Verification items for the finished model (mm, model axes). Give positions to 0.01 mm unless a question says otherwise; leave off trailing zeros. Write each loop counter-clockwise with the first axis right and the second up, starting at its lowest first coordinate (ties: lowest second). Pieces come first, ordered by that corner, then holes. Notation, with made-up numbers: (31.25, -34) -> (57.25, -34) arc R37 ccw to (57.25, 5) -> close; hole circle Ø10 at (71, 1.25). An arc over 180 degrees is marked (long way). Answer as CSV lines item,"result". Start each with the question number.
1) Mould release check, pull along Z, two halves, no side actions. Record for faces 1 (the flat face through (-6, -4, 178)), 2 (the cylindrical face through (-5.082, -5.34, 14.388)), 3 (the cylindrical face through (-0.517, 7.377, 150.747)), 4 (the flat face through (-6, -4, 0)): released by +Z, released by -Z, zero draft, split by the parting line, or undercut.
2) Sectioned sample at C-C on z = 56. Record the cut outline in (x, y).
3) Sectioned sample at B-B on z = 163. Record the cut outline in (x, y), and give its area (3 significant figures).
4) Material ranges on L1, parallel to Z at x = 0, y = 7.7; L2, parallel to Y at x = 0, z = 131.5; L3, parallel to X at y = 7.35, z = 163, recorded low to high.
5) Gauge pin test, flat ends, axial feed: pin 1 Ø6 at (y, z) = (0.5, 110.5) entering from -X; pin 2 Ø2 at (x, z) = (3.5, 119) entering from -Y; pin 3 Ø3 at (x, z) = (2, 37.5) entering from -Y. Record the tip position at first contact, or that the pin passes through.
6) Sectioned sample at A-A on y = 0. Record the cut outline in (x, z).
```python
from build123d import *

# Parameters (mm, degrees)
SKETCH1_R               = 8
SKETCH1_R_2             = 6.9
BOSS_EXTRUDE1_DEPTH     = 163
SKETCH3_R               = 8
SKETCH3_R_2             = 6.9
BOSS_EXTRUDE3_DEPTH     = 15
CUT_EXTRUDE1_DEPTH      = 179.359188157
CUT_EXTRUDE1_DEPTH_BACK = 179.359188157
SKETCH2_R               = 1.6
SKETCH2_R_2             = 1.35
SKETCH4_R               = 1.4
CUT_EXTRUDE2_DEPTH      = 179.359188267
CIRPATTERN1_COUNT       = 2
CIRPATTERN1_ANGLE       = 90


with BuildPart() as part:
    # Sketch1 → Boss-Extrude1 (new body)
    with BuildSketch(Plane.XY):
        Circle(SKETCH1_R)
        Circle(SKETCH1_R_2, mode=Mode.SUBTRACT)
    extrude(amount=BOSS_EXTRUDE1_DEPTH)

    # Sketch3 → Boss-Extrude3 (add)
    with BuildSketch(Plane.XY.offset(163)):
        Circle(SKETCH3_R)
        Circle(SKETCH3_R_2, mode=Mode.SUBTRACT)
    extrude(amount=BOSS_EXTRUDE3_DEPTH)

    # Sketch2 → Cut-Extrude1 (cut, two sides: drawn at the far end of the back side and taken through both)
    with BuildSketch(Plane(origin=(0, 0, 0), x_dir=(1, 0, 0), z_dir=(0, 1, 0)).offset(-CUT_EXTRUDE1_DEPTH_BACK)):
        with Locations(Location((0, -163, 0), (0, 0, 270))):
            Circle(SKETCH2_R)
        with Locations(Location((0, -149.5, 0), (0, 0, 270))):
            Circle(SKETCH2_R_2)
    extrude(amount=CUT_EXTRUDE1_DEPTH + CUT_EXTRUDE1_DEPTH_BACK, mode=Mode.SUBTRACT)

    # Sketch4 → Cut-Extrude2 (cut, symmetric)
    with BuildSketch(Plane(origin=(0, 0, 0), x_dir=(0, 0, 1), z_dir=(0.7071067811865464, 0.7071067811865488, 0))):
        with Locations(Location((13, 0, 0), (0, 0, 270))):
            Circle(SKETCH4_R)
        with Locations(Location((5, 0, 0), (0, 0, 270))):
            Circle(SKETCH4_R)
    cut_extrude2 = extrude(amount=CUT_EXTRUDE2_DEPTH, both=True, mode=Mode.SUBTRACT)

    # CirPattern1: Cut-Extrude2 ×2 about axis
    cirpattern1_axis = Axis((0, 0, -8.9), (0, 0, 1))
    for i in range(1, CIRPATTERN1_COUNT):
        add(cut_extrude2.rotate(cirpattern1_axis, i * CIRPATTERN1_ANGLE / (CIRPATTERN1_COUNT - 1)), mode=Mode.SUBTRACT)


solid = part.part
```
Ans:
1,face 1,"released by +Z"
1,face 2,"undercut"
1,face 3,"undercut"
1,face 4,"released by -Z"
2,outline,"circle Ø16 at (0, 0); hole circle Ø13.8 at (0, 0)"
3,outline,"(-1.6, -7.84) -> (-1.6, -6.71) arc R6.9 cw to (-1.6, 6.71) -> (-1.6, 7.84) arc R8 ccw to start; (1.6, -7.84) arc R8 ccw to (1.6, 7.84) -> (1.6, 6.71) arc R6.9 cw to (1.6, -6.71) -> close"
3,area,"44.4 mm²"
4,L1,"z = 0 to 148.15, 150.85 to 161.4, 164.6 to 178"
4,L2,"y = -8 to -6.9, 6.9 to 8"
4,L3,"x = -3.16 to -1.6, 1.6 to 3.16"
5,pin 1,"stops at x = -8"
5,pin 2,"stops at y = -7.6"
5,pin 3,"stops at y = -7.98"
6,outline,"(-8, 0) -> (-6.9, 0) -> (-6.9, 178) -> (-8, 178) -> close; (6.9, 0) -> (8, 0) -> (8, 178) -> (6.9, 178) -> close"
